Verification items for the finished model (mm, model axes). Face numbers are marked on the shaded views. A direction names the side the tool comes from. Give positions to 0.01 mm unless a question says otherwise; leave off trailing zeros. Loops run counter-clockwise (first coordinate to the right, second up) from the corner with the lowest first, then second, coordinate; pieces in that order, holes last. Notation, with made-up numbers: (52.5, 88) - (67.5, 88) arc R14 ccw to (67.5, 102) - close; hole circle Ø6 at (-1.75, -34). An arc over 180 degrees is marked (long way). One line per item, written item: value. Start each with the question number.
1. Sectioned sample at A-A (y = 35). Record the cut outline in (x, z).
2. Sectioned sample at C-C (x = -70). Record the cut outline in (y, z), plus the area to 3 significant figures.
3. Mould release check, pull along X, two halves, no side actions. Record for the marked faces 3, 4 and 5: pulls with the +X half, pulls with the -X half, needs draft (parallel to the pull), parting line crosses it, or undercut.
4. Sectioned sample at B-B (z = 37.5). Record the cut outline in (x, y).
5. Gauge pin test, flat end, axial feed: pin 1 (2 mm diameter, centred on x = -37.5, z = 48, fed in from +Y). Record the tip position at first contact, or that the pin passes through.
6. Access from +Z, -Z, +X, -X, +Y, -Y to the whole of each face (thin tool, end or side, straight path). Record for the marked faces 1 and 2.
7. Scan lines: L1, parallel to X at y = 74, z = 90.5; L2, parallel to Z at x = 63.5, y = 160; L3, parallel to Y at x = 58, z = 86.5. Record each from-to range of solid material in increasing order. Write a range as [from, to].
Autodesk Inventor part; units mm, degrees
ref_plane "YZ Plane" through (0, 0, 0) normal (1, 0, 0) x (0, 1, 0)
ref_plane "XZ Plane" through (0, 0, 0) normal (0, 1, 0) x (-1, 0, 0)
ref_plane "XY Plane" through (0, 0, 0) normal (0, 0, 1) x (1, 0, 0)
sketch "Sketch1" plane through (0, 0, 0) normal (0, 1, 0) x (-1, 0, 0)
  line L0 (-81.4912, -78.8023) -> (133.5088, -78.8023)
  line L1 (133.5088, -78.8023) -> (133.5088, 111.1977)
  line L2 (133.5088, 111.1977) -> (-81.4912, 111.1977)
  line L3 (-81.4912, 111.1977) -> (-81.4912, -78.8023)
  point P0 (0, 0)
  dimension "d0" = 190
  dimension "d1" = 215
extrude "Extrusion1" add sketch "Sketch1" along normal blind 180
sketch "Sketch2" plane through (0, 180, 0) normal (0, 1, 0) x (1, 0, 0)
  line L0 (70.7245, -100.7611) -> (-121.4246, -100.7611)
  line L1 (-121.4246, -100.7611) -> (-121.4246, 69.6594)
  line L2 (-121.4246, 69.6594) -> (70.7245, 69.6594)
  line L3 (70.7245, 69.6594) -> (70.7245, -100.7611)
  point P0 (0, 0)
extrude "Extrusion2" cut sketch "Sketch2" along normal mid plane 340
properties part number "tray2"
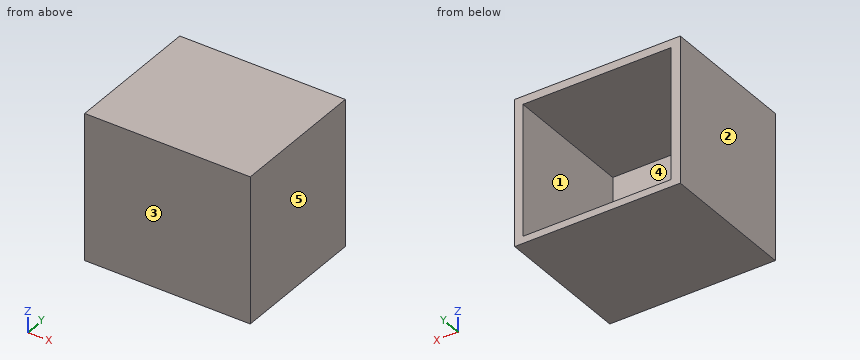
Results are:
1. outline: (-133.51, -78.8) - (81.49, -78.8) - (81.49, 111.2) - (-133.51, 111.2) - close; hole (-121.42, -69.66) - (70.72, -69.66) - (70.72, 100.76) - (-121.42, 100.76) - close
2. outline: (0, -78.8) - (180, -78.8) - (180, -69.66) - (10, -69.66) - (10, 100.76) - (180, 100.76) - (180, 111.2) - (0, 111.2) - close
2. area: 5,230 mm^2
3. face 3: needs draft
3. face 4: undercut
3. face 5: pulls with the +X half
4. outline: (-133.51, 0) - (81.49, 0) - (81.49, 180) - (70.72, 180) - (70.72, 10) - (-121.42, 10) - (-121.42, 180) - (-133.51, 180) - close
5. pin 1: stops at y = 10
6. face 1: +Y
6. face 2: +Z, -Z, -X, +Y, -Y
7. L1: x = [-133.51, -121.42], [70.72, 81.49]
7. L2: z = [-78.8, -69.66], [100.76, 111.2]
7. L3: y = [0, 10]
